Geometry check sheet. Reference: drawing and pictorial views, mm from the part's lowest x, y, z. A direction names the side the tool comes from. Give positions to 0.01 mm unless a question says otherwise; leave off trailing zeros. Loops run counter-clockwise (first coordinate to the right, second up) from the corner with the lowest first, then second, coordinate; pieces in that order, holes last. Notation, with made-up numbers: (-15.75, -11) -> (-0.75, -11) arc R10 ccw to (-0.75, -4) -> close; hole circle Ø6 at (19, -15.75). An arc over 180 degrees is marked (long way). One line per item, written item: value. Start each with the question number.
(1) Sectioned sample at B-B, the plane z = 10. Record the cut outline in (x, y).
(2) Tool access check on the marked faces 1, 2, 3, 4 and 5. Record the directions out of +Z, -Z, +X, -X, +Y, -Y that give a thin tool (end or side, any length) a straight path to the whole face; none if there is none.
(3) Sectioned sample at C-C, the plane x = 0.4. Record the cut outline in (y, z).
(4) Sectioned sample at D-D, the plane z = 18.75. Record the cut outline in (x, y), then the cut area to 3 significant figures.
(5) Gauge pin test, flat ends, axial feed: pin 1 Ø1 at (x, z) = (1.5, 2) entering from -Y; pin 2 Ø3 at (y, z) = (4.4, 10) entering from -X; pin 3 Ø1 at (x, y) = (2.5, 8) entering from +Z. Record the tip position at first contact, or that the pin passes through.
(6) Scan lines: line 1 along Y through (x, z) = (1.95, 16.25); line 2 along Z through (x, y) = (0.7, 2.5); line 3 along Z through (x, y) = (0.45, 3.5). Record each from-to range of solid material in increasing order. Write a range as from..to.
(7) Sectioned sample at A-A, the plane x = 3. Record the cut outline in (y, z), then the cut area to 3 significant figures.
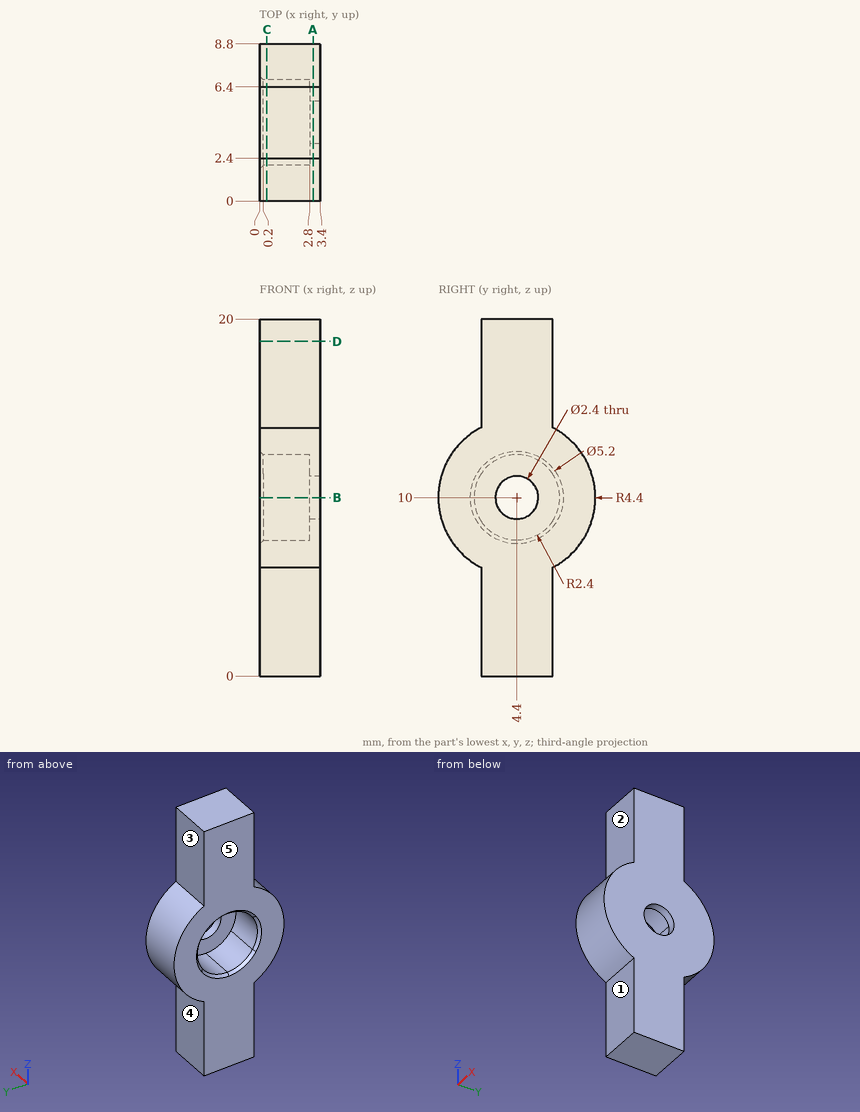
Calculated:
1. outline: (0, 0) -> (3.4, 0) -> (3.4, 3.2) -> (2.8, 3.2) -> (2.8, 2) -> (0.2, 2) -> (0, 1.8) -> close; (0, 7) -> (0.2, 6.8) -> (2.8, 6.8) -> (2.8, 5.6) -> (3.4, 5.6) -> (3.4, 8.8) -> (0, 8.8) -> close
2. face 1: -Z, +X, -X, -Y
2. face 2: +Z, +X, -X, -Y
2. face 3: +Z, +X, -X, +Y
2. face 4: -Z, +X, -X, +Y
2. face 5: +Z, -Z, -X, +Y, -Y
3. outline: (2.4, 0) -> (6.4, 0) -> (6.4, 6.08) arc R4.4 ccw to (6.4, 13.92) -> (6.4, 20) -> (2.4, 20) -> (2.4, 13.92) arc R4.4 ccw to (2.4, 6.08) -> close; hole circle Ø4.8 at (4.4, 10)
4. outline: (0, 2.4) -> (3.4, 2.4) -> (3.4, 6.4) -> (0, 6.4) -> close
4. area: 13.6 mm2
5. pin 1: stops at y = 2.4
5. pin 2: stops at x = 2.8
5. pin 3: stops at z = 13.12
6. line 1: y = 2.4..6.4
6. line 2: z = 0..8.53, 11.47..20
6. line 3: z = 0..7.78, 12.22..20
7. outline: (2.4, 0) -> (6.4, 0) -> (6.4, 6.08) arc R4.4 ccw to (6.4, 13.92) -> (6.4, 20) -> (2.4, 20) -> (2.4, 13.92) arc R4.4 ccw to (2.4, 6.08) -> close; hole circle Ø2.4 at (4.4, 10)
7. area: 102 mm2
